Could you check a few things on this model? Use its own coordinates, in mm. A direction names the side the tool comes from. Give positions to 0.01 mm unless a question says otherwise; leave off trailing zeros. Loops run counter-clockwise (first coordinate to the right, second up) from the corner with the lowest first, then second, coordinate; pieces in that order, holes last. Notation, with made-up numbers: M 60.25,43 L 107.25,43 A32 cw 107.25,71 Z; hole C 72,-36.5 d2. An arc over 180 degrees is marked long. Return JSON: item names as keys, results as strings. Group by question number.
1. For pin 1 (5 mm diameter, centred on x = -7, y = -1, fed in from -Z); pin 2 (1.5 mm diameter, centred on x = -2, z = 1.5, fed in from -Y), each with a flat end and sliding along its axis, tell me the tip position at first contact or that it passes through.
2. If we section it at A-A (y = -11.5): Write out the boundary of the cut face in (x, z), plus the area to 4 significant figures.
3. Please list where these lines run through material, in increasing order: line 1 (X direction, y = -10, z = 0.5); line 2 (Y direction, x = 3.25, z = 8.5); line 3 (Z direction, x = -7.75, y = -18).
4. If we section it at B-B (z = 5): Write out the boundary of the cut face in (x, y).
5. If we mould it in two halves opening along Y, with no side actions, what happens to faces 4 (the flat face through (-7.2, -2.1, 0)), 5 (the flat face through (-3, 10.305, 5)), 6 (the flat face through (-9, -7, 7.25))? For each: +Y half, -Y half, draft (parallel to the pull), parting line (faces both ways), or undercut.
6. If we section it at D-D (y = 4): Write out the boundary of the cut face in (x, z).
7. If we section it at C-C (x = -8): Write out the boundary of the cut face in (y, z), plus the area to 3 significant figures.
8. For faces 1 (the flat face through (-7.005, -8, 2)), 2 (the cylindrical face through (-8.678, 5.555, 5.049)), 3 (the flat face through (4.895, 9, 5)), which set-ups out of +Z, -Z, +X, -X, +Y, -Y let a thin tool reach every point of the face, with its end or its side?
```python
from build123d import *

# Parameters (mm, degrees)
BOSS_EXTRUDE1_DEPTH = 10
CUT_EXTRUDE1_DEPTH  = 6


with BuildPart() as part:
    # Sketch1 → Boss-Extrude1 (new body)
    with BuildSketch(Plane.XY):
        Polygon((-10.305084746, -21.694915254), (-7.005084746, -21.694915254), (-7.005084746, 7.005084746), (4.894915254, 7.005084746), (4.894915254, 10.305084746), (-10.305084746, 10.305084746), align=None)
    extrude(amount=BOSS_EXTRUDE1_DEPTH)

    # Sketch2 → Cut-Extrude1 (cut)
    with BuildSketch(Plane.ZY.offset(10.305084746)):
        with BuildLine():
            Line((2.75, 3.305084746), (2.75, -17.694915254))
            ThreePointArc((2.75, -17.694915254), (5, -19.944915254), (7.25, -17.694915254))
            Line((7.25, -17.694915254), (7.25, 3.305084746))
            ThreePointArc((7.25, 3.305084746), (5, 5.555084746), (2.75, 3.305084746))
        make_face()
    extrude(amount=-CUT_EXTRUDE1_DEPTH, mode=Mode.SUBTRACT)


solid = part.part
```
Answer:
{
 "1": {"pin 1": "stops at z = 0", "pin 2": "stops at y = 7.01"},
 "2": {"outline": "M -10.31,0 L -7.01,0 L -7.01,2.75 L -10.31,2.75 Z; M -10.31,7.25 L -7.01,7.25 L -7.01,10 L -10.31,10 Z", "area": "18.15 mm²"},
 "3": {"line 1": "x = -10.31 to -7.01", "line 2": "y = 7.01 to 10.31", "line 3": "z = 0 to 2.77, 7.23 to 10"},
 "4": {"outline": "M -10.31,-21.69 L -7.01,-21.69 L -7.01,-19.94 L -10.31,-19.94 Z; M -10.31,5.56 L -7.01,5.56 L -7.01,7.01 L 4.89,7.01 L 4.89,10.31 L -10.31,10.31 Z"},
 "5": {"face 4": "draft", "face 5": "+Y half", "face 6": "undercut"},
 "6": {"outline": "M -10.31,0 L -7.01,0 L -7.01,2.86 L -10.31,2.86 Z; M -10.31,7.14 L -7.01,7.14 L -7.01,10 L -10.31,10 Z"},
 "7": {"outline": "M -21.69,0 L 10.31,0 L 10.31,10 L -21.69,10 Z; hole M -17.69,2.75 L 3.31,2.75 A2.25 ccw 3.31,7.25 L -17.69,7.25 A2.25 ccw Z", "area": "210 mm²"},
 "8": {"face 1": "+Z, -Z, +X, -Y", "face 2": "+X, -X", "face 3": "+Z, -Z, +X, +Y, -Y"}
}
